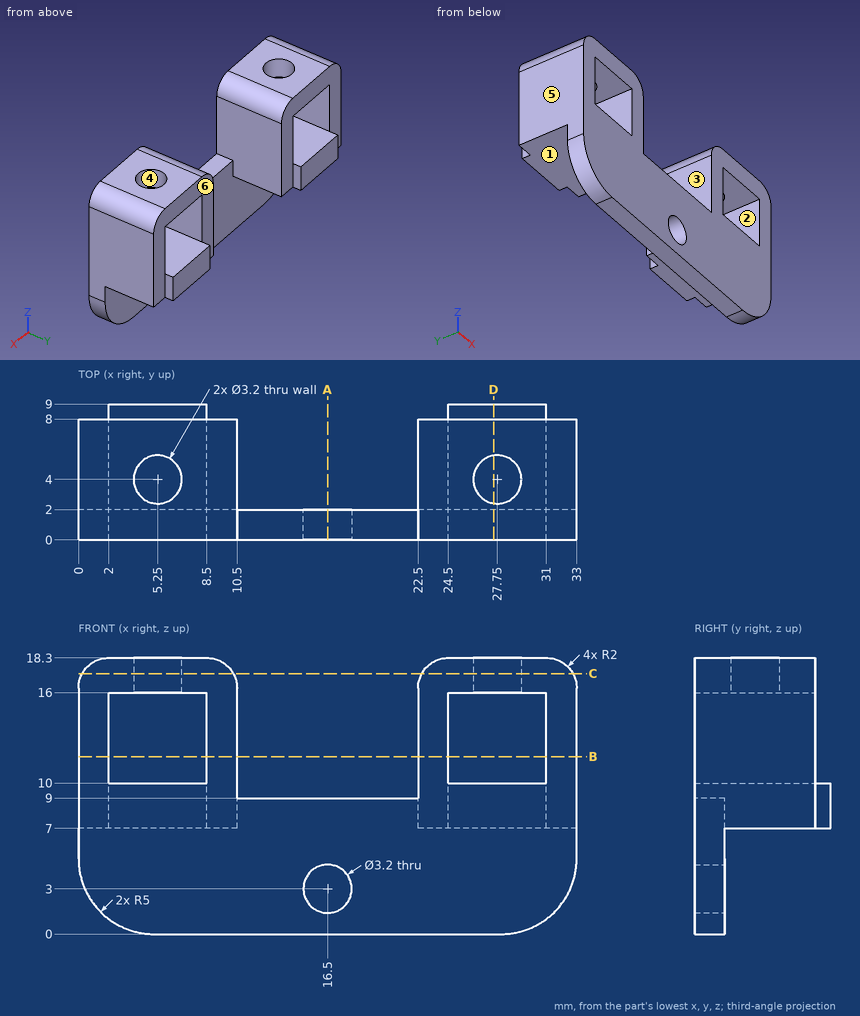
The figure shows three views and two pictorial views of one solid part (mm, origin at its lowest corner). Answer the questions. A direction names the side the tool comes from. Round coordinates to 2 decimals unless told otherwise and drop trailing zeros. Order: outer loops, then holes, each group sorted by start corner. A loop starts at its lowest first (then second) coordinate and runs counter-clockwise, first axis right, second up. Notation, with made-up numbers: (-8, 59) - (49, 59) arc R19 cw to (49, 87) - close; hole circle Ø1 at (35, -29.75). An arc over 180 degrees is marked (long way). Write item = value, one per line. Start each with the question number.
1) Straight lines are drawn through the part: L1, parallel to Z at x = 16.5, y = 0.4; L2, parallel to X at y = 5.5, z = 7.25; L3, parallel to Y at x = 27.75, z = 16.95. For each, find the intervals that lie inside material, in ascending order.
2) Section D-D, the plane x = 27.5 is taken. Write down the section's boundary in (y, z).
3) Section B-B, the plane z = 11.75 is taken. Write down the section's boundary in (x, y), plus the area to 3 significant figures.
4) Section C-C, the plane z = 17.25 is taken. Write down the section's boundary in (x, y), plus the area to 3 significant figures.
5) Section A-A, the plane x = 16.5 is taken. Write down the section's boundary in (y, z), plus the area to 3 significant figures.
6) For the marked faces 1, 2 and 3, determine the directions among +Z, -Z, +X, -X, +Y, -Y from which every point of the face is accessible in a straight line to the end or side of a thin tool.
7) For a pull along Y with two mould halves and no side action, classify the marked faces 4, 5 and 6 as released by +Y, released by -Y, zero draft, split by the parting line, or undercut.
8) Given pin 1 (2 mm diameter, centred on x = 28.5, y = 4, fed in from -Z); pin 2 (1.6 mm diameter, centred on x = 16.5, y = 0.5, fed in from +Z); pin 3 (10 mm diameter, centred on x = 14, z = 4, fed in from +Y), each flat-ended and moving along its own axis, determine where each tip first touches the part or whether it passes through.
Results list:
q1.L1 = 0 to 1.4, 4.6 to 9
q1.L2 = 0 to 10.5, 22.5 to 33
q1.L3 = 0 to 2.4, 5.6 to 8
q2.outline = (0, 0) - (2, 0) - (2, 7) - (9, 7) - (9, 10) - (0, 10) - close; (0, 16) - (2.42, 16) - (2.42, 18.3) - (0, 18.3) - close; (5.58, 16) - (8, 16) - (8, 18.3) - (5.58, 18.3) - close
q3.outline = (0, 0) - (2, 0) - (2, 8) - (0, 8) - close; (8.5, 0) - (10.5, 0) - (10.5, 8) - (8.5, 8) - close; (22.5, 0) - (24.5, 0) - (24.5, 8) - (22.5, 8) - close; (31, 0) - (33, 0) - (33, 8) - (31, 8) - close
q3.area = 64.0 mm^2
q4.outline = (0.24, 0) - (10.26, 0) - (10.26, 8) - (0.24, 8) - close; (22.74, 0) - (32.76, 0) - (32.76, 8) - (22.74, 8) - close; hole circle Ø3.2 at (5.25, 4); hole circle Ø3.2 at (27.75, 4)
q4.area = 144 mm^2
q5.outline = (0, 0) - (2, 0) - (2, 1.4) - (0, 1.4) - close; (0, 4.6) - (2, 4.6) - (2, 9) - (0, 9) - close
q5.area = 11.6 mm^2
q6.face_1 = -Z, +X, -X, +Y
q6.face_2 = +Y, -Y
q6.face_3 = +Z, +Y
q7.face_4 = undercut
q7.face_5 = zero draft
q7.face_6 = released by +Y
q8.pin_1 = 7
q8.pin_2 = 9
q8.pin_3 = 8
